Could you check a few things on this model? Use its own coordinates, in mm. Face numbers are marked on the shaded views. A direction names the side the tool comes from. Coordinates: 2 decimals unless noted, no trailing zeros. Order: outer loops, then holes, each group sorted by start corner. A loop starts at its lowest first (then second) coordinate and runs counter-clockwise, first axis right, second up. Notation, with made-up numbers: (47, 2) - (56, 2) arc R30 ccw to (56, 25) - close; hole circle Ø1 at (26, 46.5). An arc over 180 degrees is marked (long way). One line per item, written item: value.
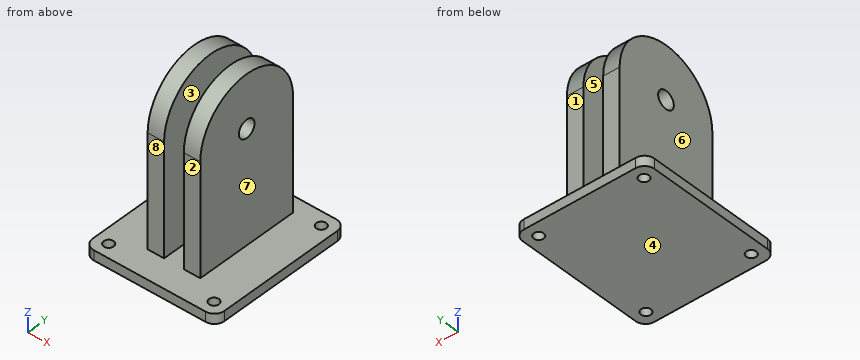
from build123d import *

# Parameters (mm, degrees)
SKETCH1_W           = 40
SKETCH1_H           = 45
BOSS_EXTRUDE1_DEPTH = 3
SKETCH2_W           = 5
SKETCH2_H           = 32
BOSS_EXTRUDE2_DEPTH = 50
SKETCH3_R           = 2.7
CUT_EXTRUDE1_DEPTH  = 451.662125067
FILLET2_R           = 3
SKETCH4_R           = 1.5
CUT_EXTRUDE2_DEPTH  = 450.892599372


with BuildPart() as part:
    # Sketch1 → Boss-Extrude1 (new body)
    with BuildSketch(Plane.XY):
        with Locations((0, 424.157979857)):
            Rectangle(SKETCH1_W, SKETCH1_H)
    extrude(amount=BOSS_EXTRUDE1_DEPTH)

    # Sketch2 → Boss-Extrude2 (add)
    with BuildSketch(Plane.XY.offset(3)):
        with Locations((5.5, 426)):
            Rectangle(SKETCH2_W, SKETCH2_H)
        with Locations((-5.5, 426)):
            Rectangle(SKETCH2_W, SKETCH2_H)
    extrude(amount=BOSS_EXTRUDE2_DEPTH)

    # Sketch3 → Cut-Extrude1 (cut, through all)
    with BuildSketch(Plane(origin=(8, 0, 0), x_dir=(0, 0, -1), z_dir=(1, 0, 0))):
        with Locations(Location((-37, 426, 0), (0, 0, 90))):
            Circle(SKETCH3_R)
        with BuildLine():
            Line((-37, 442), (-57.90422328, 442))
            Line((-57.90422328, 442), (-57.90422328, 410))
            Line((-57.90422328, 410), (-37, 410))
            ThreePointArc((-37, 410), (-53, 426), (-37, 442))
        make_face()
    extrude(amount=-CUT_EXTRUDE1_DEPTH, mode=Mode.SUBTRACT)

    # Fillet2
    fillet2_edges = [part.edges().sort_by_distance(p)[0] for p in [
        (-20, 446.657979857, 1.5),
        (20, 446.657979857, 1.5),
        (20, 401.657979857, 1.5),
        (-20, 401.657979857, 1.5),
    ]]
    fillet(fillet2_edges, radius=FILLET2_R)

    # Sketch4 → Cut-Extrude2 (cut, through all)
    with BuildSketch(Plane.XY.offset(3)):
        with Locations((-16, 442.657979857)):
            Circle(SKETCH4_R)
        with Locations(Location((-16, 405.657979857, 0), (0, 0, 180))):
            Circle(SKETCH4_R)
        with Locations((16, 405.657979857)):
            Circle(SKETCH4_R)
        with Locations(Location((16, 442.657979857, 0), (0, 0, 180))):
            Circle(SKETCH4_R)
    extrude(amount=-CUT_EXTRUDE2_DEPTH, mode=Mode.SUBTRACT)


solid = part.part
Item 1: I want a section at D-D on y = 421. Please give me the cut outline in (x, z), then the cut area to 3 significant figures.
Conclusion:
outline: (-20, 0) - (20, 0) - (20, 3) - (8, 3) - (8, 52.2) - (3, 52.2) - (3, 3) - (-3, 3) - (-3, 52.2) - (-8, 52.2) - (-8, 3) - (-20, 3) - close
area: 612 mm²
Item 2: I want a section at C-C on x = 16. Please give me the cut outline in (y, z).
Conclusion:
outline: (401.66, 0) - (404.16, 0) - (404.16, 3) - (401.66, 3) - close; (407.16, 0) - (441.16, 0) - (441.16, 3) - (407.16, 3) - close; (444.16, 0) - (446.66, 0) - (446.66, 3) - (444.16, 3) - close
Item 3: Thinking about a two-plate mould opening in X: for the marked faces 5, 6, 7 and 8, which applies, pulls with the +X half, pulls with the -X half, needs draft (parallel to the pull), parting line crosses it, or undercut?
Conclusion:
face 5: undercut
face 6: pulls with the -X half
face 7: pulls with the +X half
face 8: needs draft
Item 4: If I drill on probe 1 along Y at (x, z) = (16, 1.5); probe 2 along X at (y, z) = (412.5, 10.5); probe 3 along Z at (x, y) = (-1.5, 432), over which ranges is the centre line in solid material (lowest first)?
Conclusion:
probe 1: 401.66 to 404.16, 407.16 to 441.16, 444.16 to 446.66
probe 2: -8 to -3, 3 to 8
probe 3: 0 to 3
Item 5: For the marked faces 1, 2, 3 and 4, which set-ups out of +Z, -Z, +X, -X, +Y, -Y let a thin tool reach every point of the face, with its end or its side?
Conclusion:
face 1: +Z, +X, -X, +Y
face 2: +Z, +X, -X, -Y
face 3: +Z, +Y, -Y
face 4: -Z, +X, -X, +Y, -Y
Item 6: I want a section at A-A on z = 27. Please give me the cut outline in (x, y).
Conclusion:
outline: (-8, 410) - (-3, 410) - (-3, 442) - (-8, 442) - close; (3, 410) - (8, 410) - (8, 442) - (3, 442) - close
Item 7: I'm going to push flat-ended pins straight in: pin 1 Ø1.5 at (x, z) = (-4.5, 25) entering from -Y; pin 2 Ø5 at (x, z) = (12.5, 42) entering from +Y; pin 3 Ø1 at (y, z) = (412.5, 6.5) entering from -X; pin 4 Ø10 at (y, z) = (408, 27.5) entering from +X. Where does each tip first touch, or does it pass through?
Conclusion:
pin 1: y = 410
pin 2: through
pin 3: x = -8
pin 4: x = 8
Item 8: I want a section at B-B on x = -6. Please give me the cut outline in (y, z).
Conclusion:
outline: (401.66, 0) - (446.66, 0) - (446.66, 3) - (442, 3) - (442, 37) arc R16 ccw to (410, 37) - (410, 3) - (401.66, 3) - close; hole circle Ø5.4 at (426, 37)
